Work out the finished part from the listing and answer in its coordinate system (mm). Face numbers are marked on the shaded views. A direction names the side the tool comes from. Round coordinates to 2 decimals unless told otherwise and drop trailing zeros. Loops run counter-clockwise (first coordinate to the right, second up) from the corner with the lowest first, then second, coordinate; pieces in that order, holes last. Notation, with made-up numbers: (-10, -8.5) - (38, -8.5) arc R23 cw to (38, 2.5) - close; hole circle Ø1 at (-0.75, -1). An arc over 180 degrees is marked (long way). Answer as CSV lines item,"result". Start each with the question number.
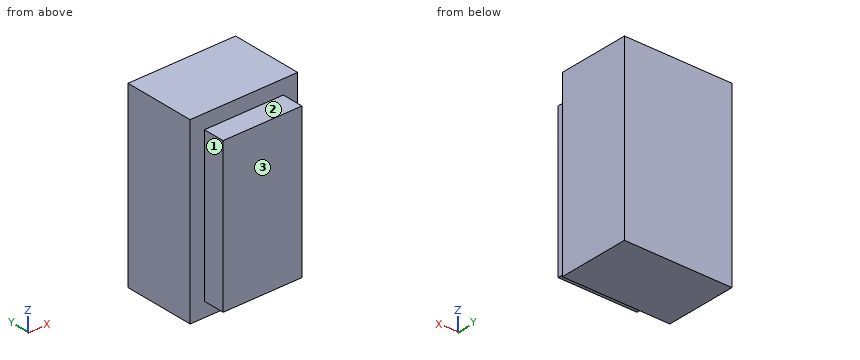
```python
from build123d import *

# Parameters (mm, degrees)
BOX025_W                  = 11
BOX025_H                  = 7
BOX025_DEPTH              = 21
BOX024_W                  = 15
BOX024_H                  = 10
BOX024_DEPTH              = 25
FUSION005_PLACEMENT_ANGLE = 180


with BuildPart() as box025:
    # Box025 → Box025 (new body)
    with BuildSketch(Plane(origin=(227, 236, 227), x_dir=(1, 0, 0), z_dir=(0, 0, 1))):
        with Locations((5.5, 3.5)):
            Rectangle(BOX025_W, BOX025_H)
    extrude(amount=BOX025_DEPTH)


with BuildPart() as ac_plug_switch:
    # Box024 → Box024 (new body)
    with BuildSketch(Plane(origin=(225, 230, 225), x_dir=(1, 0, 0), z_dir=(0, 0, 1))):
        with Locations((7.5, 5)):
            Rectangle(BOX024_W, BOX024_H)
    extrude(amount=BOX024_DEPTH)

    # Fusion005: union Box025
    add(box025.part)


with BuildPart() as ac_plug_switch_1:
    # Fusion005 placement: moved
    add(ac_plug_switch.part.moved(Location((510, 238, -90))).rotate(Axis((510, 238, -90), (0, 0, 1)), FUSION005_PLACEMENT_ANGLE))


solid = ac_plug_switch_1.part
```
Item 1: Flat-ended cylindrical pins translate along their axes: pin 1 Ø0.9 at (x, y) = (276.5, -3.5) entering from +Z; pin 2 Ø2.5 at (y, z) = (-4, 146.5) entering from +X; pin 3 Ø1.5 at (x, y) = (279, -4) entering from -Z. Find the tip coordinate at first contact, or state that the pin passes through.
Item 2: Section B-B, the plane z = 148.25 is taken. Give the vertices of the cut face in (x, y), and give its area (3 significant figures).
Item 3: Which of the six approach directions +Z, -Z, +X, -X, +Y, -Y give full straight-line access (tool end or side, diameter ignored) to the marked faces 1, 2 and 3?
Item 4: Section A-A, the plane x = 280 is taken. Give the vertices of the cut face in (y, z).
Item 5: Section D-D, the plane x = 283.75 is taken. Give the vertices of the cut face in (y, z).
Item 6: Find the intervals of material crossed by L1, parallel to Z at x = 279, y = -2.5; L2, parallel to X at y = -3, z = 142.5; L3, parallel to Y at x = 283.75, z = 143.5, in increasing order.
Item 7: Section C-C, the plane y = -2.75 is taken. Give the vertices of the cut face in (x, z), and give its area (3 significant figures).
Answer:
1,pin 1,"stops at z = 158"
1,pin 2,"stops at x = 283"
1,pin 3,"stops at z = 137"
2,outline,"(270, -2) - (272, -2) - (272, -5) - (283, -5) - (283, -2) - (285, -2) - (285, 8) - (270, 8) - close"
2,area,"183 mm²"
3,face 1,"+Z, -Z, -X, -Y"
3,face 2,"+Z, +X, -X, -Y"
3,face 3,"+Z, -Z, +X, -X, -Y"
4,outline,"(-5, 137) - (-2, 137) - (-2, 135) - (8, 135) - (8, 160) - (-2, 160) - (-2, 158) - (-5, 158) - close"
5,outline,"(-2, 135) - (8, 135) - (8, 160) - (-2, 160) - close"
6,L1,"z = 137 to 158"
6,L2,"x = 272 to 283"
6,L3,"y = -2 to 8"
7,outline,"(272, 137) - (283, 137) - (283, 158) - (272, 158) - close"
7,area,"231 mm²"
